Work out the finished part from the listing and answer in its coordinate system (mm). A direction names the side the tool comes from. Give positions to 0.01 mm unless a question says otherwise; leave off trailing zeros. Loops run counter-clockwise (first coordinate to the right, second up) from the corner with the lowest first, then second, coordinate; pieces in that order, holes last. Notation, with made-up numbers: (47, -1) - (96, -1) arc R22 cw to (96, 14) - close; hole circle Ø4 at (-30.75, -26.75). An arc over 180 degrees is marked (long way). One line per item, written item: value.
from build123d import *

# Parameters (mm, degrees)
SKETCH1_R                              = 22.5
SKETCH1_R_2                            = 12.5
BOSS_EXTRUDE1_DEPTH                    = 35
BOSS_EXTRUDE2_START                    = 10
SKETCH2_R                              = 45
SKETCH2_R_2                            = 12.5
BOSS_EXTRUDE2_DEPTH                    = 10
CUT_EXTRUDE1_START                     = 11
CUT_EXTRUDE1_DEPTH                     = 5.500000008
CUT_EXTRUDE1_START_2                   = -33
CUT_EXTRUDE1_2_DEPTH                   = 32
CBORE_FOR_M6_HEX_HEAD_BOLT1_AT_2_COUNT = 2
CBORE_FOR_M6_HEX_HEAD_BOLT1_AT_2_PITCH = 49.497474683
CBORE_FOR_M6_HEX_HEAD_BOLT1_AT_3_COUNT = 2
CBORE_FOR_M6_HEX_HEAD_BOLT1_AT_3_PITCH = 70
CBORE_FOR_M6_HEX_HEAD_BOLT1_AT_4_COUNT = 2
CBORE_FOR_M6_HEX_HEAD_BOLT1_AT_4_PITCH = 49.497474683


with BuildPart() as part:
    # Sketch1 → Boss-Extrude1 (new body)
    with BuildSketch(Plane.XY):
        Circle(SKETCH1_R)
        Circle(SKETCH1_R_2, mode=Mode.SUBTRACT)
    extrude(amount=-BOSS_EXTRUDE1_DEPTH)

    # Sketch2 → Boss-Extrude2 (add)
    with BuildSketch(Plane.XY.offset(BOSS_EXTRUDE2_START)):
        Circle(SKETCH2_R)
        Circle(SKETCH2_R_2, mode=Mode.SUBTRACT)
    extrude(amount=-BOSS_EXTRUDE2_DEPTH)

    # Cut-Extrude1: read off the stored shape, not the designer's step
    # Cut-Extrude1 outline → Cut-Extrude1 (cut)
    with BuildSketch(Plane(origin=(0, 0, 0), x_dir=(1, 0, 0), z_dir=(0, 1, 0)).offset(CUT_EXTRUDE1_START)):
        with BuildLine():
            add(Edge.make_bspline(
                [(-4, 28), (-4, 29.064380904), (-3.561099342, 30.095615587), (-2.096292766, 31.560700753), (-1.055346498, 31.998914356), (1.04710073, 32.001081394), (2.090364215, 31.566087585), (3.564946316, 30.092309962), (4, 29.064475319), (4, 28)],
                knots=[0, 0, 0, 0, 0.25, 0.25, 0.5, 0.5, 0.75, 0.75, 1, 1, 1, 1], degree=3))
            Line((-4, 28), (-4, 6))
            add(Edge.make_bspline(
                [(4, 6), (4, 4.935619096), (3.561099342, 3.904384413), (2.096292766, 2.439299247), (1.055346498, 2.001085644), (-1.04710073, 1.998918606), (-2.090364215, 2.433912415), (-3.564946316, 3.907690038), (-4, 4.935524681), (-4, 6)],
                knots=[0, 0, 0, 0, 0.25, 0.25, 0.5, 0.5, 0.75, 0.75, 1, 1, 1, 1], degree=3))
            Line((4, 6), (4, 28))
        make_face()
    extrude(amount=CUT_EXTRUDE1_DEPTH, mode=Mode.SUBTRACT)

    # Cut-Extrude1 2 outline → Cut-Extrude1 2 (add)
    with BuildSketch(Plane.XY.offset(CUT_EXTRUDE1_START_2)):
        with BuildLine():
            ThreePointArc((-4, 15.842719282), (-2.026821151, 16.334585361), (2.53e-07, 16.5))
            Line((2.53e-07, 16.5), (-4, 16.500000008))
            Line((-4, 16.500000008), (-4, 15.842719282))
        make_face()
        with BuildLine():
            ThreePointArc((2.53e-07, 16.5), (2.026821401, 16.33458532), (4, 15.842719282))
            Line((4, 15.842719282), (4, 16.500000008))
            Line((4, 16.500000008), (2.53e-07, 16.5))
        make_face()
    extrude(amount=CUT_EXTRUDE1_2_DEPTH)

    # Sketch5 → CBORE for M6 Hex Head Bolt1 (revolve, cut)
    with BuildSketch(Plane.YZ.offset(35)):
        Polygon((0, 0), (0, 10), (3.2, 10), (3.2, 4.38), (7.275, 4.38), (7.275, 0.025), (7.3, 0), align=None)
    cbore_for_m6_hex_head_bolt1 = revolve(axis=Axis((35, 0, -6.35), (0, 0, 1)), mode=Mode.SUBTRACT)

    # CBORE for M6 Hex Head Bolt1 at 2: CBORE for M6 Hex Head Bolt1 ×2
    with Locations(*[Vector(-0.7071067811865512, 0.7071067811865438, 0) * (i * CBORE_FOR_M6_HEX_HEAD_BOLT1_AT_2_PITCH) for i in range(1, CBORE_FOR_M6_HEX_HEAD_BOLT1_AT_2_COUNT)]):
        add(cbore_for_m6_hex_head_bolt1, mode=Mode.SUBTRACT)

    # CBORE for M6 Hex Head Bolt1 at 3: CBORE for M6 Hex Head Bolt1 ×2
    with Locations(*[(-i * CBORE_FOR_M6_HEX_HEAD_BOLT1_AT_3_PITCH, 0, 0) for i in range(1, CBORE_FOR_M6_HEX_HEAD_BOLT1_AT_3_COUNT)]):
        add(cbore_for_m6_hex_head_bolt1, mode=Mode.SUBTRACT)

    # CBORE for M6 Hex Head Bolt1 at 4: CBORE for M6 Hex Head Bolt1 ×2
    with Locations(*[Vector(-0.7071067811865414, -0.7071067811865538, 0) * (i * CBORE_FOR_M6_HEX_HEAD_BOLT1_AT_4_PITCH) for i in range(1, CBORE_FOR_M6_HEX_HEAD_BOLT1_AT_4_COUNT)]):
        add(cbore_for_m6_hex_head_bolt1, mode=Mode.SUBTRACT)


solid = part.part
1. Section C-C (z = -11.5) is taken. Write down the section's boundary in (x, y).
Output:
outline: circle Ø45 at (0, 0); hole (-4, 11.84) arc R12.5 ccw (long way) to (4, 11.84) - (4, 15.84) arc R12.5 ccw to (-4, 15.84) - close
2. The mould has two halves that part along X. Classify faces 1 (the flat face through (38, -2, 4.38)), 2 (the flat face through (3, -37, 4.38)), 3 (the cylindrical face through (20.765, -39.923, 5.07)), 4 (the flat face through (10, -10, -35)): released by +X, released by -X, zero draft, split by the parting line, or undercut.
Output:
face 1: undercut
face 2: undercut
face 3: split by the parting line
face 4: zero draft
3. Section B-B (x = -35) is taken. Write down the section's boundary in (y, z) (3 decimals).
Output:
outline: (-28.284, 0) - (-7.3, 0) - (-7.275, 0.025) - (-7.275, 4.38) - (-3.2, 4.38) - (-3.2, 10) - (-28.284, 10) - close; (3.2, 4.38) - (7.275, 4.38) - (7.275, 0.025) - (7.3, 0) - (28.284, 0) - (28.284, 10) - (3.2, 10) - close
4. Flat-ended cylindrical pins translate along their axes: pin 1 Ø4 at (x, z) = (-20.5, -1) entering from -Y; pin 2 Ø20 at (x, y) = (0, 0) entering from -Z; pin 3 Ø13 at (x, y) = (-35, 0) entering from -Z; pin 4 Ø1.5 at (y, z) = (11, -6) entering from +X. Find the tip coordinate at first contact, or state that the pin passes through.
Output:
pin 1: stops at y = -40.9
pin 2: passes through
pin 3: stops at z = 4.38
pin 4: stops at x = 20.03
5. Find the intervals of material crossed by line 1 along Z through (x, y) = (-27.5, 26); line 2 along X through (y, z) = (1, -16.5); line 3 along X through (y, z) = (-3, -22), in increasing order.
Output:
line 1: z = 0 to 10
line 2: x = -22.48 to -12.46, 12.46 to 22.48
line 3: x = -22.3 to -12.13, 12.13 to 22.3
6. Section A-A (y = 0) is taken. Count the separate pieces of the cut face and the enclosed holes in it, and give its area (3 significant figures).
Output:
separate pieces: 4
enclosed holes: 0
area: 1,150 mm²
7. For faces 5 (the cylindrical face through (-38.173, -0.417, 7.151)), 6 (the flat face through (4, 14, -17)), 7 (the flat face through (-32, -2, 4.38)), determine the directions among +Z, -Z, +X, -X, +Y, -Y from which every point of the face is accessible in a straight line to the end or side of a thin tool.
Output:
face 5: +Z, -Z
face 6: none
face 7: -Z
